For this review, take the finished solid that the model builds, in its own axes (mm). A direction names the side the tool comes from. Coordinates: 2 decimals unless noted, no trailing zeros. Write each loop counter-clockwise with the first axis right and the second up, starting at its lowest first coordinate (ties: lowest second). Pieces come first, ordered by that corner, then holes.
Autodesk Inventor part; units mm, degrees
ref_plane "YZ Plane" through (0, 0, 0) normal (1, 0, 0) x (0, 1, 0)
ref_plane "XZ Plane" through (0, 0, 0) normal (0, 1, 0) x (-1, 0, 0)
ref_plane "XY Plane" through (0, 0, 0) normal (0, 0, 1) x (1, 0, 0)
sketch "スケッチ1" plane through (0, 0, 0) normal (0, 0, 1) x (1, 0, 0)
  line L0 (0, 0) -> (110, 0)
  line L1 (110, 0) -> (110, 20)
  line L2 (110, 20) -> (0, 20)
  line L3 (0, 20) -> (0, 0)
  dimension "d0" = 110
  dimension "d1" = 20
extrude "押し出し1" add sketch "スケッチ1" along normal blind 5
sketch "スケッチ2" plane through (0, 0, 0) normal (0, 0, -1) x (-1, 0, 0)
  line L0 (-110, 0) -> (-110, 20)
  line L1 (0, 0) -> (-110, 0)
  line L2 (0, 20) -> (0, 0)
  line L3 (-110, 20) -> (0, 20)
  line L4 (-2.5, 20) -> (-7.5, 20)
  line L5 (-7.5, 20) -> (-7.5, 0)
  line L6 (-7.5, 0) -> (-2.5, 0)
  line L7 (-2.5, 0) -> (-2.5, 20)
  line L8 (-107.5, 0) -> (-102.5, 0)
  line L9 (-102.5, 0) -> (-102.5, 20)
  line L10 (-102.5, 20) -> (-107.5, 20)
  line L11 (-107.5, 20) -> (-107.5, 0)
  point P0 (-107.5, 20)
  point P1 (-102.5, 0)
  dimension "d4" = 5
  dimension "d5" = 2.5
  dimension "d6" = 5
  dimension "d7" = 2.5
extrude "押し出し2" cut sketch "スケッチ2" against normal blind 1 contours L11 L3 L9 L1 | L5 L3 L7 L1
sketch "スケッチ3" plane through (0, 0, 5) normal (0, -1, 0) x (1, 0, 0)
  line L0 (30.22, -4) -> (25.22, -4)
  line L1 (25.22, -4) -> (25.22, -356)
  line L2 (25.22, -356) -> (30.22, -356)
  line L3 (30.22, -356) -> (30.22, -4)
extrude "押し出し3" cut sketch "スケッチ3" against normal through all
properties part number "arm1_S"
Q1. Add section A-A (y = 12.25). State the section outline as (x, z) points.
Ans:
outline: (0, 0) - (2.5, 0) - (2.5, 1) - (7.5, 1) - (7.5, 0) - (25.22, 0) - (25.22, 1) - (30.22, 1) - (30.22, 0) - (102.5, 0) - (102.5, 1) - (107.5, 1) - (107.5, 0) - (110, 0) - (110, 5) - (0, 5) - close
Q2. Tool access review of faces 1 (the flat face through (109, 10, 0)), 2 (the flat face through (5, 10, 1)): name each direction out of +Z, -Z, +X, -X, +Y, -Y from which nothing blocks a thin tool from reaching the whole face with its end or side.
Ans:
face 1: -Z, +X, -X, +Y, -Y
face 2: -Z, +Y, -Y
Q3. Clearance check with a flat-ended pin moving along its axis: pin 1 Ø2.5 at (x, y) = (5, 6) entering from -Z. State where the tip first meets the part, or that it passes through.
Ans:
pin 1: stops at z = 1
Q4. For probe 1 along Z at (x, y) = (30, 16), list the stretches that pass through material, from the lowest coordinate up.
Ans:
probe 1: z = 1 to 5
Q5. Draft analysis for pull direction X (two halves, no side actions). For faces 3 (the flat face through (105, 10, 1)), 4 (the flat face through (110, 10, 2)), 5 (the flat face through (28, 10, 1)), 6 (the flat face through (54, 0, 2)), state which applies: +X half, -X half, draft (parallel to the pull), parting line (faces both ways), or undercut.
Ans:
face 3: undercut
face 4: +X half
face 5: undercut
face 6: draft
